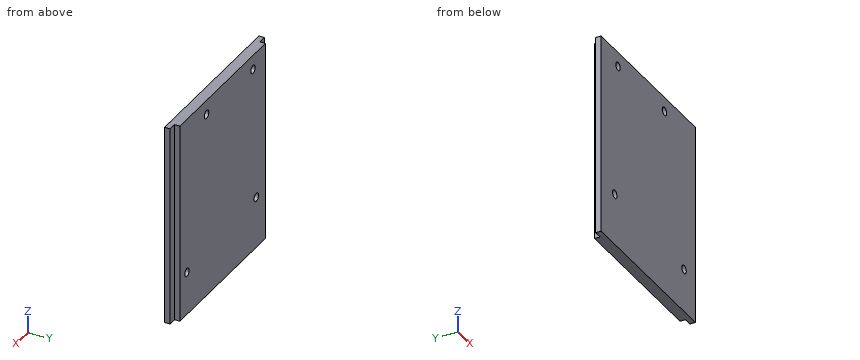
Autodesk Inventor part; units mm, degrees
ref_plane "YZ Plane" through (0, 0, 0) normal (1, 0, 0) x (0, 1, 0)
ref_plane "XZ Plane" through (0, 0, 0) normal (0, 1, 0) x (-1, 0, 0)
ref_plane "XY Plane" through (0, 0, 0) normal (0, 0, 1) x (1, 0, 0)
sketch "Sketch1" plane through (0, 0, 0) normal (0, 1, 0) x (-1, 0, 0)
  line L0 (0, 0) -> (-53.5, 0)
  line L1 (-53.5, 0) -> (-53.5, -68.5)
  line L2 (-53.5, -68.5) -> (0, -68.5)
  line L3 (0, -68.5) -> (0, 0)
  dimension "d0" = 53.5
  dimension "d1" = 68.5
extrude "Extrusion1" add sketch "Sketch1" along normal blind 4
sketch "Sketch2" plane through (0, 4, 0) normal (0, 1, 0) x (1, 0, 0)
  circle A0 centre (51, 55.0126) radius 1.5
  line L0 (53.5, 68.5) -> (0, 68.5)
  line L1 (53.5, 0) -> (53.5, 68.5)
  circle A1 centre (4, 52) radius 1.5
  line L2 (0, 68.5) -> (0, 0)
  circle A2 centre (37.7012, 3) radius 1.5
  line L3 (0, 0) -> (53.5, 0)
  circle A3 centre (6.223, 3) radius 1.5
  dimension "d4" = 3
  dimension "d5" = 13.4874
  dimension "d6" = 2.5
  dimension "d7" = 3
  dimension "d8" = 16.5
  dimension "d9" = 4
  dimension "d10" = 3
  dimension "d11" = 15.7988
  dimension "d12" = 3
  dimension "d13" = 3
  dimension "d14" = 3
  dimension "d15" = 6.223
extrude "Extrusion2" cut sketch "Sketch2" against normal blind 12 contours A0 | A1 | A2 | A3
sketch "Sketch3" plane through (0, 4, 0) normal (0, 1, 0) x (1, 0, 0)
  line L0 (0, 0) -> (53.5, 0)
  line L1 (53.5, 0) -> (53.5, 68.5)
  line L2 (53.5, 68.5) -> (0, 68.5)
  line L3 (0, 68.5) -> (0, 0)
  line L4 (-2.25, -2.25) -> (55.75, -2.25)
  line L5 (55.75, -2.25) -> (55.75, 70.75)
  line L6 (55.75, 70.75) -> (-2.25, 70.75)
  line L7 (-2.25, 70.75) -> (-2.25, -2.25)
  dimension "d18" = 2.25
extrude "Extrusion3" add sketch "Sketch3" against normal blind 4
sketch "Sketch6" plane through (55.75, 4, 2.25) normal (1, 0, 0) x (0, 0, -1)
  line L0 (0, 0) -> (73, 0)
  line L1 (73, -4) -> (0, -4)
  line L2 (0, 0) -> (73, 0)
  line L3 (0, 0) -> (0, -4)
  line L4 (73, -4) -> (0, -4)
  line L5 (73, 0) -> (73, -4)
  line L6 (73, 0) -> (73, -4)
  line L7 (0, -4) -> (73, -4)
  line L8 (73, -4) -> (73, -2)
  line L9 (73, -2) -> (0, -2)
  line L10 (0, -2) -> (0, -4)
  point P0 (2.25, -4)
  dimension "d33" = 2
extrude "Extrusion6" add sketch "Sketch6" along normal blind 3 contours L9 L5 L1 L3
sketch "Sketch7" plane through (-2.25, 4, -70.75) normal (-1, 0, 0) x (0, 0, 1)
  line L0 (73, -4) -> (0, -4)
  line L1 (0, -4) -> (0, -2)
  line L2 (0, -2) -> (73, -2)
  line L3 (73, -2) -> (73, -4)
  point P0 (70.75, -4)
extrude "Extrusion7" add sketch "Sketch7" along normal blind 3
properties part number "uno-holder"
Can you work these out from the model? Positions are in its coordinate system, mm. Coordinates: 2 decimals unless noted, no trailing zeros. Loops run counter-clockwise (first coordinate to the right, second up) from the corner with the lowest first, then second, coordinate; pieces in that order, holes last.
1) I need wall thicknesses on probe 1 along X at (y, z) = (2.75, -3); probe 2 along Z at (x, y) = (37.5, 1.6); probe 3 along X at (y, z) = (1.25, -52). Which ranges of each line are inside material? Lowest first, please.
2) For pin 1 (1 mm diameter, centred on y = 3, z = -38, fed in from -X); pin 2 (3 mm diameter, centred on x = 6.5, z = -40, fed in from -Y); pin 3 (1.6 mm diameter, centred on y = 3.5, z = -49, fed in from +X); pin 4 (0.9 mm diameter, centred on x = 56.5, z = -48.5, fed in from +Y), each with a flat end and sliding along its axis, tell me the tip position at first contact or that it passes through.
3) Imagine slicing it at A-A on x = 51. List the corners of the cut face in (y, z) for me.
4) Imagine slicing it at B-B on z = -52. List the corners of the cut face in (x, y) for me.
5) Imagine slicing it at D-D on y = 3.05. List the corners of the cut face in (x, z) for me, plus the area to 3 significant figures.
6) Imagine slicing it at C-C on z = -3. List the corners of the cut face in (x, y) for me, plus the area to 3 significant figures.
Completed:
1. probe 1: x = -2.25 to 4.72, 7.72 to 36.2, 39.2 to 55.75
1. probe 2: z = -70.75 to -4.49, -1.51 to 2.25
1. probe 3: x = -5.25 to 2.5, 5.5 to 58.75
2. pin 1: stops at x = -2.25
2. pin 2: stops at y = 0
2. pin 3: stops at x = 55.75
2. pin 4: stops at y = 2
3. outline: (0, -70.75) - (4, -70.75) - (4, -56.51) - (0, -56.51) - close; (0, -53.51) - (4, -53.51) - (4, 2.25) - (0, 2.25) - close
4. outline: (-5.25, 0) - (2.5, 0) - (2.5, 4) - (-2.25, 4) - (-2.25, 2) - (-5.25, 2) - close; (5.5, 0) - (58.75, 0) - (58.75, 2) - (55.75, 2) - (55.75, 4) - (5.5, 4) - close
5. outline: (-2.25, -70.75) - (55.75, -70.75) - (55.75, 2.25) - (-2.25, 2.25) - close; hole circle Ø3 at (4, -52); hole circle Ø3 at (6.22, -3); hole circle Ø3 at (37.7, -3); hole circle Ø3 at (51, -55.01)
5. area: 4,210 mm2
6. outline: (-5.25, 0) - (4.72, 0) - (4.72, 4) - (-2.25, 4) - (-2.25, 2) - (-5.25, 2) - close; (7.72, 0) - (36.2, 0) - (36.2, 4) - (7.72, 4) - close; (39.2, 0) - (58.75, 0) - (58.75, 2) - (55.75, 2) - (55.75, 4) - (39.2, 4) - close
6. area: 220 mm2
